The listing builds one solid part. Answer for the finished solid, in the listing's coordinates (mm). Face numbers are marked on the shaded views. A direction names the side the tool comes from. Give positions to 0.01 mm unless a question says otherwise; leave off trailing zeros. Order: outer loops, then holes, each group sorted by start corner. A loop starts at its lowest first (then second) coordinate and runs counter-clockwise, first axis right, second up.
```python
from build123d import *

# Parameters (mm, degrees)
F1_DEPTH = 25.4
F2_R     = 13.3061005932
F3_DEPTH = 25.401
F5_DEPTH = 25.401
F6_W     = 52.0203243941
F6_H     = 47.6390495896
F7_DEPTH = 25.4
F8_W     = 26.2038465589
F8_H     = 14.3460799009
F9_DEPTH = 25.4


with BuildPart() as f1:
    # F0 (on Top) → F1 (new body)
    with BuildSketch(Plane.XY):
        with BuildLine():
            Line((-25.3657195717, 48.8345064223), (25.3657195717, 48.8345064223))
            ThreePointArc((25.3657195717, 48.8345064223), (0, 74.200225994), (-25.3657195717, 48.8345064223))
        make_face()
        with BuildLine():
            Line((25.3657195717, 0), (25.3657195717, 48.8345064223))
            ThreePointArc((25.3657195717, 48.8345064223), (0, 23.4687868506), (-25.3657195717, 48.8345064223))
            Line((-25.3657195717, 48.8345064223), (-25.3657195717, 0))
            Line((-25.3657195717, 0), (25.3657195717, 0))
        make_face()
        with BuildLine():
            ThreePointArc((-25.3657195717, 48.8345064223), (0, 23.4687868506), (25.3657195717, 48.8345064223))
            Line((25.3657195717, 48.8345064223), (-25.3657195717, 48.8345064223))
        make_face()
    extrude(amount=F1_DEPTH)

    # F2 (on Top) → F3 (cut, through all)
    with BuildSketch(Plane.XY):
        with Locations((0, 48.2391826808)):
            Circle(F2_R)
    extrude(amount=F3_DEPTH, mode=Mode.SUBTRACT)

    # F2 (on Top) → F5 (cut, through all)
    with BuildSketch(Plane.XY):
        with Locations((0, 48.2391826808)):
            Circle(F2_R)
    extrude(amount=F5_DEPTH, mode=Mode.SUBTRACT)

    # F6 (on Front) → F7 (join)
    with BuildSketch(Plane.XZ):
        with Locations((0.1023123041, 23.8195247948)):
            Rectangle(F6_W, F6_H)
    extrude(amount=F7_DEPTH)

    # F8 (on Front) → F9 (cut)
    with BuildSketch(Plane.XZ):
        with Locations((13.1019232795, 41.2792069837)):
            Rectangle(F8_W, F8_H)
    extrude(amount=F9_DEPTH, mode=Mode.SUBTRACT)


solid = f1.part
```
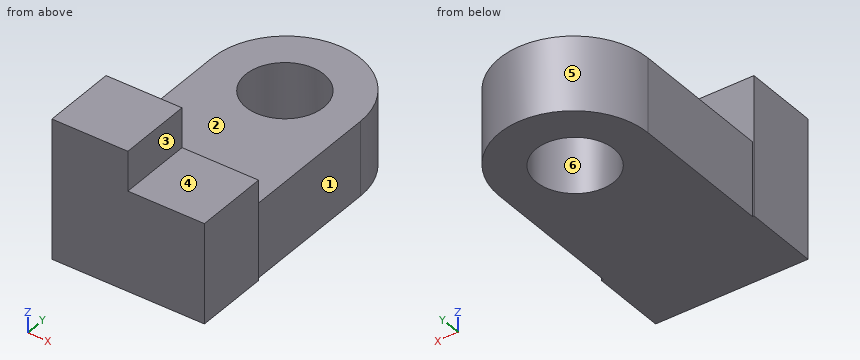
1) Find section D-D (z = 3). Write down the section's boundary in (x, y), then the cut area to 3 significant figures.
Geometry says:
outline: (-25.91, -25.4) - (26.11, -25.4) - (26.11, 0) - (25.37, 0) - (25.37, 48.83) arc R25.37 ccw to (-25.37, 48.83) - (-25.37, 0) - (-25.91, 0) - close; hole circle Ø26.61 at (0, 48.24)
area: 4,250 mm2
2) A tool of negligible diameter and unlimited length cuts with its end or side. For the marked faces 1, 2 and 3, from which of +Z, -Z, +X, -X, +Y, -Y can it reach the whole face along a straight path? Write none if from no direction.
Geometry says:
face 1: +Z, -Z, +X, +Y
face 2: +Z, +X, -X, +Y
face 3: +Z, +X, +Y, -Y
3) For a pull along X with two mould halves and no side action, classify the marked faces 4, 5 and 6 as +X half, -X half, draft (parallel to the pull), parting line (faces both ways), or undercut.
Geometry says:
face 4: draft
face 5: parting line
face 6: undercut
4) Straight lines are drawn through the part: probe 1 along Y at (x, z) = (0, 10.25); probe 2 along X at (y, z) = (-5, 37); probe 3 along Z at (x, y) = (-20, 21.5). For each, find the intervals that lie inside material, in ascending order.
Geometry says:
probe 1: y = -25.4 to 34.93, 61.55 to 74.2
probe 2: x = -25.91 to 0
probe 3: z = 0 to 25.4
5) Find section A-A (y = 36). Write down the section's boundary in (x, z).
Geometry says:
outline: (-25.37, 0) - (-5.22, 0) - (-5.22, 25.4) - (-25.37, 25.4) - close; (5.22, 0) - (25.37, 0) - (25.37, 25.4) - (5.22, 25.4) - close
6) Find section C-C (y = -6.5). Write down the section's boundary in (x, z), then the cut area to 3 significant figures.
Geometry says:
outline: (-25.91, 0) - (26.11, 0) - (26.11, 34.11) - (0, 34.11) - (0, 47.64) - (-25.91, 47.64) - close
area: 2,120 mm2
7) Find section B-B (x = -6). Write down the section's boundary in (y, z), then the cut area to 3 significant figures.
Geometry says:
outline: (-25.4, 0) - (36.36, 0) - (36.36, 25.4) - (0, 25.4) - (0, 47.64) - (-25.4, 47.64) - close; (60.12, 0) - (73.48, 0) - (73.48, 25.4) - (60.12, 25.4) - close
area: 2,470 mm2
8) Given P1, Ø5, axis at x = -1.5, z = 10.5, coming from the +Y side; P2, Ø6, axis at x = 17, y = -5.5, coming from the +Z side; P3, Ø4, axis at x = 15.5, z = 27, coming from the +Y side, each flat-ended and moving along its own axis, determine where each tip first touches the part or whether it passes through.
Geometry says:
P1: stops at y = 74.2
P2: stops at z = 34.11
P3: stops at y = 69.79
